Check sheet for the modelled part. Datum: model origin and axes. Units: mm. Give positions to 0.01 mm unless a question says otherwise; leave off trailing zeros. Order: outer loops, then holes, each group sorted by start corner. A loop starts at its lowest first (then second) coordinate and runs counter-clockwise, first axis right, second up.
Item 1: Gauge pin test, flat ends, axial feed: P1, Ø4, axis at y = -185.5, z = 4.5, coming from the +X side; P2, Ø5, axis at x = 0, z = 0, coming from the -Y side; P3, Ø14.5, axis at x = 0, z = 0, coming from the -Y side. Record the tip position at first contact, or that the pin passes through.
Item 2: Sectioned sample at B-B on y = -42. Record the boundary of the cut face in (x, z), and give its area (3 significant figures).
Item 3: Material ranges on line 1 along Y through (x, z) = (20.5, 13.5); line 2 along Z through (x, y) = (0, -355); line 3 along X through (y, z) = (-366, 0), recorded low to high.
Item 4: Sectioned sample at A-A on y = -262. Record the boundary of the cut face in (x, z).
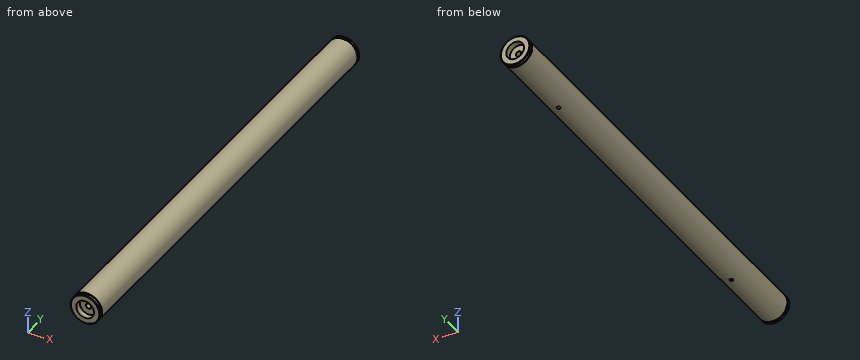
from build123d import *

# Parameters (mm, degrees)
SKETCH_1_R                = 25
EXTRUDE_1_DEPTH           = 373
SKETCH_2_R                = 15
CUT_EXTRUDE_1_DEPTH       = 10
HOLE_WIZARD_8_0_8_1_D     = 8
HOLE_WIZARD_8_0_8_1_DEPTH = 119
HOLE_WIZARD_8_0_8_1_TIP   = 2.403442476
SKETCH_5_R                = 3
CUT_EXTRUDE_2_DEPTH       = 100
M10X1_0_1_D               = 9
M10X1_0_1_DEPTH           = 25
M10X1_0_1_TIP             = 2.703872786
CUT_EXTRUDE_START         = -10
SKETCH_8_R                = 15
CUT_EXTRUDE_3_DEPTH       = 10
HOLE_WIZARD_8_0_8_2_D     = 8
HOLE_WIZARD_8_0_8_2_DEPTH = 119
HOLE_WIZARD_8_0_8_2_TIP   = 2.403442476
M10X1_0_2_D               = 9
M10X1_0_2_DEPTH           = 25
M10X1_0_2_TIP             = 2.703872786
SKETCH_12_R               = 3
CUT_EXTRUDE_4_DEPTH       = 51
CHAMFER_1_SIZE            = 1
SKETCH_14_W               = 1.5
SKETCH_14_H               = 2.2


with BuildPart() as part:
    # 草图1 → 凸台-拉伸1 (new, symmetric)
    with BuildSketch(Plane(origin=(0, 0, 0), x_dir=(1, 0, 0), z_dir=(0, 1, 0))):
        with Locations(Location((0, 0, 0), (0, 0, 270))):
            Circle(SKETCH_1_R)
    extrude(amount=EXTRUDE_1_DEPTH, both=True)

    # 草图2 → 切除-拉伸1 (cut)
    with BuildSketch(Plane(origin=(0, 373, 0), x_dir=(1, 0, 0), z_dir=(0, 1, 0))):
        with Locations(Location((0, 0, 0), (0, 0, 270))):
            Circle(SKETCH_2_R)
    extrude(amount=-CUT_EXTRUDE_1_DEPTH, mode=Mode.SUBTRACT)

    # Ø8.0 (8) 直径孔1
    with Locations(Plane.ZX.offset(363)):
        with Locations((0, 0)):
            Hole(HOLE_WIZARD_8_0_8_1_D / 2, depth=HOLE_WIZARD_8_0_8_1_DEPTH)
            with Locations((0, 0, -(HOLE_WIZARD_8_0_8_1_DEPTH + HOLE_WIZARD_8_0_8_1_TIP / 2))):  # 118° drill point
                Cone(0, HOLE_WIZARD_8_0_8_1_D / 2, HOLE_WIZARD_8_0_8_1_TIP, mode=Mode.SUBTRACT)

    # 草图5 → 切除-拉伸2 (cut)
    with BuildSketch(Plane.XY):
        with Locations((0, 248)):
            Circle(SKETCH_5_R)
    extrude(amount=-CUT_EXTRUDE_2_DEPTH, mode=Mode.SUBTRACT)

    # M10x1.0 螺纹孔1
    with Locations(Plane(origin=(0, 363, 0), x_dir=(1, 0, 0), z_dir=(0, 1, 0))):
        with Locations((0, 0)):
            Hole(M10X1_0_1_D / 2, depth=M10X1_0_1_DEPTH)
            with Locations((0, 0, -(M10X1_0_1_DEPTH + M10X1_0_1_TIP / 2))):  # 118° drill point
                Cone(0, M10X1_0_1_D / 2, M10X1_0_1_TIP, mode=Mode.SUBTRACT)

    # 草图8 → 切除-拉伸3 (cut)
    with BuildSketch(Plane.XZ.offset(373).offset(CUT_EXTRUDE_START)):
        with Locations(Location((0, 0, 0), (0, 0, 90))):
            Circle(SKETCH_8_R)
    extrude(amount=CUT_EXTRUDE_3_DEPTH, mode=Mode.SUBTRACT)

    # Ø8.0 (8) 直径孔2
    with Locations(Plane(origin=(0, -363, 0), x_dir=(0, 0, -1), z_dir=(0, -1, 0))):
        with Locations((0, 0)):
            Hole(HOLE_WIZARD_8_0_8_2_D / 2, depth=HOLE_WIZARD_8_0_8_2_DEPTH)
            with Locations((0, 0, -(HOLE_WIZARD_8_0_8_2_DEPTH + HOLE_WIZARD_8_0_8_2_TIP / 2))):  # 118° drill point
                Cone(0, HOLE_WIZARD_8_0_8_2_D / 2, HOLE_WIZARD_8_0_8_2_TIP, mode=Mode.SUBTRACT)

    # M10x1.0 螺纹孔2
    with Locations(Plane(origin=(0, -363, 0), x_dir=(-1, 0, 0), z_dir=(0, -1, 0))):
        with Locations((0, 0)):
            Hole(M10X1_0_2_D / 2, depth=M10X1_0_2_DEPTH)
            with Locations((0, 0, -(M10X1_0_2_DEPTH + M10X1_0_2_TIP / 2))):  # 118° drill point
                Cone(0, M10X1_0_2_D / 2, M10X1_0_2_TIP, mode=Mode.SUBTRACT)

    # 草图12 → 切除-拉伸4 (cut)
    with BuildSketch(Plane.XY):
        with Locations(Location((0, -248, 0), (0, 0, 90))):
            Circle(SKETCH_12_R)
    extrude(amount=-CUT_EXTRUDE_4_DEPTH, mode=Mode.SUBTRACT)

    # 倒角1
    chamfer_1_edges = [part.edges().sort_by_distance(p)[0] for p in [
        (0, -373, -25),
        (0, 373, -25),
    ]]
    chamfer(chamfer_1_edges, length=CHAMFER_1_SIZE)

    # 草图14 → 切除-旋转1 (revolve, cut)
    with BuildSketch(Plane(origin=(0, 0, 0), x_dir=(0, 0, -1), z_dir=(1, 0, 0))):
        with Locations((24.25, 367.4)):
            Rectangle(SKETCH_14_W, SKETCH_14_H)
        with Locations((24.25, -367.4)):
            Rectangle(SKETCH_14_W, SKETCH_14_H)
    revolve(axis=Axis((0, 0, 0), (0, 1, 0)), mode=Mode.SUBTRACT)


solid = part.part
Report:
1. P1: stops at x = 24.87
1. P2: stops at y = -243.1
1. P3: stops at y = -363
2. outline: circle Ø50 at (0, 0)
2. area: 1,960 mm2
3. line 1: y = -372.45 to -368.5, -366.3 to 366.3, 368.5 to 372.45
3. line 2: z = -25 to -4.5, 4.5 to 25
3. line 3: x = -25 to -15, 15 to 25
4. outline: circle Ø50 at (0, 0); hole circle Ø8 at (0, 0)
